Autodesk Inventor part; units mm, degrees
ref_plane "YZ Plane" through (0, 0, 0) normal (1, 0, 0) x (0, 1, 0)
ref_plane "XZ Plane" through (0, 0, 0) normal (0, 1, 0) x (-1, 0, 0)
ref_plane "XY Plane" through (0, 0, 0) normal (0, 0, 1) x (1, 0, 0)
sketch "Sketch1" plane through (0, 0, 0) normal (0, 0, 1) x (1, 0, 0)
  circle A0 centre (0, 0) radius 15
extrude "Extrusion1" add sketch "Sketch1" along normal blind 30
chamfer "Chamfer1" distance 3 angle 45 1 edges at (-15, 0, 30)
sketch "Sketch2" plane through (0, 0, 30) normal (0, 0, 1) x (1, 0, 0)
  circle A0 centre (0, 0) radius 2
extrude "Extrusion2" add sketch "Sketch2" along normal blind 4
sketch "Sketch3" plane through (0, 0, 34) normal (0, 0, 1) x (1, 0, 0)
  circle A0 centre (0, 0) radius 1.5
extrude "Extrusion3" add sketch "Sketch3" along normal blind 8
fillet "Fillet1" radius 1 2 edges at (-2, 0, 34) (-1.5, 0, 34)
sketch "Sketch4" plane through (0, 0, 30) normal (0, 0, 1) x (1, 0, 0)
  point P0 (0, 0)
sketch "Sketch5" plane through (0, 0, 30) normal (0, 0, 1) x (1, 0, 0)
  circle A0 centre (0, 0) radius 12
  circle A1 centre (6.5184, -6.551) radius 1.25
  circle A2 centre (-6.3094, 6.5625) radius 1.25
  circle A3 centre (6.5184, 6.5625) radius 1.25
  circle A4 centre (-6.4741, -6.551) radius 1.25
extrude "Extrusion4" cut sketch "Sketch5" against normal blind 8 contours A1 | A2 | A3 | A4
sketch "Sketch6" plane through (0, 0, 0) normal (0, 0, -1) x (-1, 0, 0)
  point P0 (0, 0)
hole "Hole1" at (0, 0, 0) direction (0, 0, 1) diameter 4 depth 10 tip angle 120
properties part number "DCMotorv2"
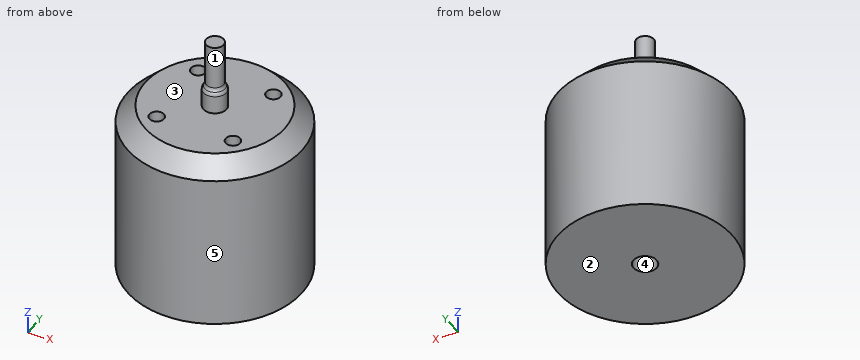
The listing builds one solid part. Answer for the finished solid, in the listing's coordinates (mm). Face numbers are marked on the shaded views. A direction names the side the tool comes from. Give positions to 0.01 mm unless a question says otherwise; leave off trailing zeros. Order: outer loops, then holes, each group sorted by start corner. A loop starts at its lowest first (then second) coordinate and runs counter-clockwise, first axis right, second up. Notation, with made-up numbers: (46, 23) -> (105, 23) arc R29 cw to (105, 44) -> close; hole circle Ø4 at (29.5, 48). An arc over 180 degrees is marked (long way). One line per item, written item: value.
1) Determine the mould class of the marked faces 3, 4 and 5 for opening direction Y: pulls with the +Y half, pulls with the -Y half, needs draft (parallel to the pull), parting line crosses it, or undercut.
Reported:
face 3: needs draft
face 4: undercut
face 5: parting line crosses it
2) A tool of negligible diameter and unlimited length cuts with its end or side. For the marked faces 1 and 2, from which of +Z, -Z, +X, -X, +Y, -Y can it reach the whole face along a straight path? Write none if from no direction.
Reported:
face 1: +Z
face 2: -Z, +X, -X, +Y, -Y
3) Find section B-B, the plane z = 29. Determine the outline of the cut face in (x, y).
Reported:
outline: circle Ø26 at (0, 0); hole circle Ø2.5 at (-6.47, -6.55); hole circle Ø2.5 at (-6.31, 6.56); hole circle Ø2.5 at (6.52, -6.55); hole circle Ø2.5 at (6.52, 6.56)
4) Find the intervals of material crossed by line 1 (X direction, y = -6.25, z = 28); line 2 (Z direction, x = 7.5, y = -2.75); line 3 (X direction, y = -5.5, z = 15.5), in increasing order.
Reported:
line 1: x = -12.53 to -7.69, -5.26 to 5.31, 7.73 to 12.53
line 2: z = 0 to 30
line 3: x = -13.96 to 13.96
5) Find section A-A, the plane z = 7.5. Determine the outline of the cut face in (x, y).
Reported:
outline: circle Ø30 at (0, 0); hole circle Ø4 at (0, 0)
6) Find section C-C, the plane z = 35.5. Determine the outline of the cut face in (x, y), plus the area to 3 significant figures.
Reported:
outline: circle Ø3 at (0, 0)
area: 7.07 mm^2
7) Flat-ended cylindrical pins translate along their axes: P1, Ø3, axis at x = 6.52, y = -6.55, coming from the +Z side; P2, Ø4, axis at x = -7, z = 14.5, coming from the -Y side; P3, Ø5, axis at y = -4, z = 23.5, coming from the +X side. Find the tip coordinate at first contact, or state that the pin passes through.
Reported:
P1: stops at z = 30
P2: stops at y = -14.14
P3: stops at x = 14.92
